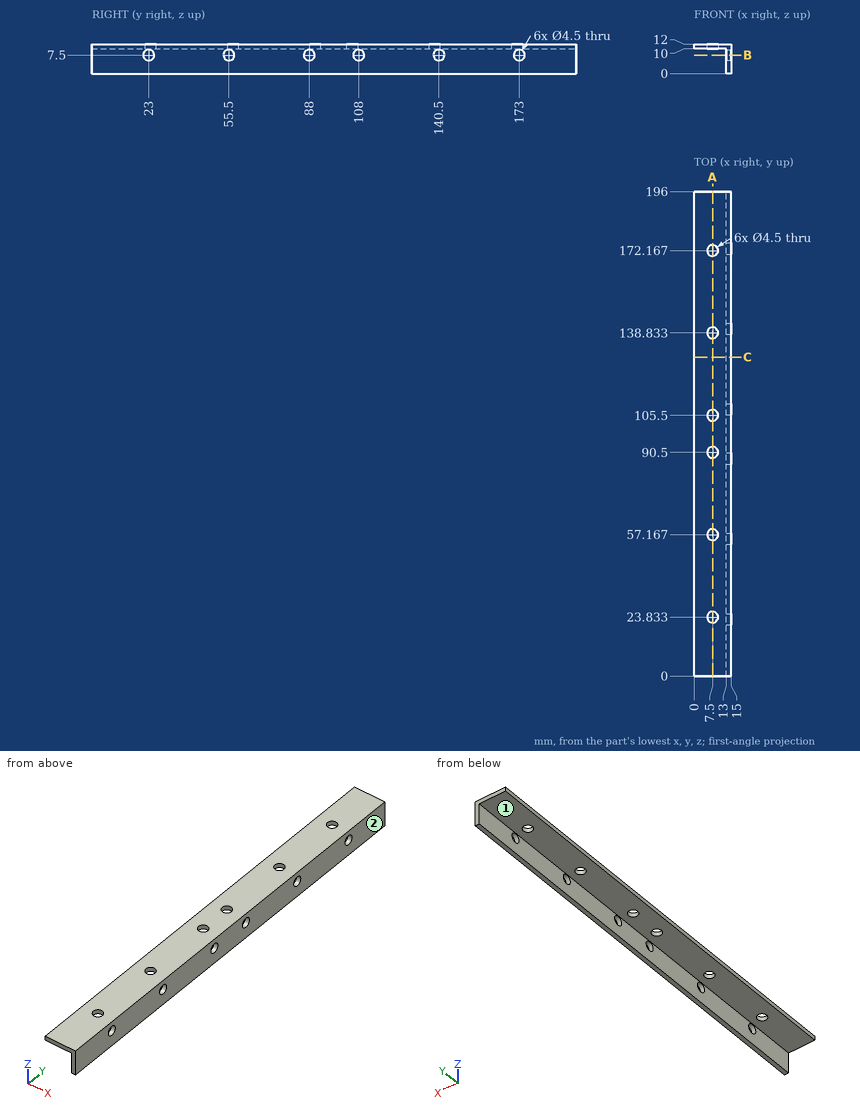
Drawing for the job (mm, zero at the part's lowest x, y, z). A direction names the side the tool comes from. Give positions to 0.01 mm unless a question says otherwise; leave off trailing zeros. Loops run counter-clockwise (first coordinate to the right, second up) from the corner with the lowest first, then second, coordinate; pieces in that order, holes last.
(1) Band-saw the part on C-C (y = 129). Write the cut outline in (x, z), and give its area (3 significant figures).
Return value:
outline: (0, 10) - (13, 10) - (13, 0) - (15, 0) - (15, 12) - (0, 12) - close
area: 50.0 mm2
(2) Band-saw the part on B-B (z = 7.5). Write the cut outline in (x, y).
Return value:
outline: (13, 0) - (15, 0) - (15, 20.75) - (13, 20.75) - close; (13, 25.25) - (15, 25.25) - (15, 53.25) - (13, 53.25) - close; (13, 57.75) - (15, 57.75) - (15, 85.75) - (13, 85.75) - close; (13, 90.25) - (15, 90.25) - (15, 105.75) - (13, 105.75) - close; (13, 110.25) - (15, 110.25) - (15, 138.25) - (13, 138.25) - close; (13, 142.75) - (15, 142.75) - (15, 170.75) - (13, 170.75) - close; (13, 175.25) - (15, 175.25) - (15, 196) - (13, 196) - close
(3) Drill centre lines: line 1 along Z through (x, y) = (8.5, 85); line 2 along X through (y, z) = (171, 5.5); line 3 along X through (y, z) = (137.5, 10.75). Where is each one in solid material? Low to high.
Return value:
line 1: z = 10 to 12
line 2: x = 13 to 15
line 3: x = 0 to 5.69, 9.31 to 15
(4) Band-saw the part on A-A (x = 7.5). Write the cut outline in (y, z).
Return value:
outline: (0, 10) - (21.58, 10) - (21.58, 12) - (0, 12) - close; (26.08, 10) - (54.92, 10) - (54.92, 12) - (26.08, 12) - close; (59.42, 10) - (88.25, 10) - (88.25, 12) - (59.42, 12) - close; (92.75, 10) - (103.25, 10) - (103.25, 12) - (92.75, 12) - close; (107.75, 10) - (136.58, 10) - (136.58, 12) - (107.75, 12) - close; (141.08, 10) - (169.92, 10) - (169.92, 12) - (141.08, 12) - close; (174.42, 10) - (196, 10) - (196, 12) - (174.42, 12) - close
(5) 3-axis set-ups, long thin cutter, end or side, ignore diameter. For the marked faces 1 and 2: which of +Z, -Z, +X, -X, +Y, -Y reach the whole face in a straight line?
Return value:
face 1: -Z, -X, +Y, -Y
face 2: +Z, -Z, +X, +Y, -Y
(6) Pin check, flat tip, straight feed: pin 1 (3 mm diameter, centred on y = 110, z = 8, fed in from -X). Stop position of the tip, or through.
Return value:
pin 1: stops at x = 13
